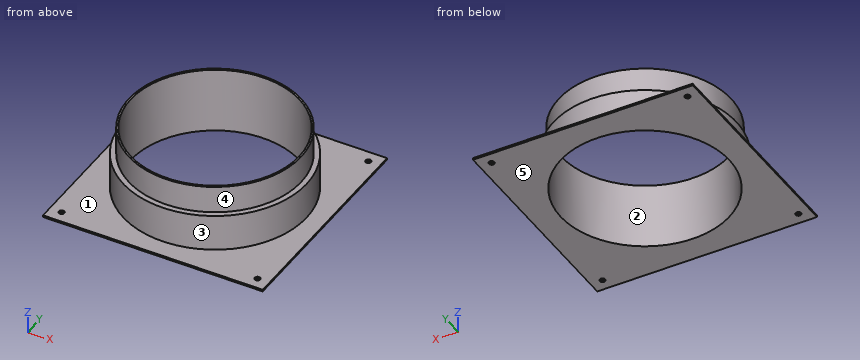
```python
from build123d import *

# Parameters (mm, degrees)
F0_W     = 120
F0_H     = 120
F1_DEPTH = 1
F2_R     = 50
F3_DEPTH = 20
F4_R     = 47
F5_DEPTH = 15
F6_R     = 46
F7_DEPTH = 56.8
F8_R     = 1.5
F9_DEPTH = 25


with BuildPart() as f1:
    # F0 (on Top) → F1 (new body)
    with BuildSketch(Plane.XY):
        Rectangle(F0_W, F0_H)
    extrude(amount=F1_DEPTH)

    # F2 (on face) → F3 (join)
    with BuildSketch(Plane.XY.offset(1)):
        Circle(F2_R)
    extrude(amount=F3_DEPTH)

    # F4 (on face) → F5 (join)
    with BuildSketch(Plane.XY.offset(21)):
        Circle(F4_R)
    extrude(amount=F5_DEPTH)

    # F6 (on face) → F7 (cut)
    with BuildSketch(Plane.XY.offset(36)):
        Circle(F6_R)
    extrude(amount=-F7_DEPTH, mode=Mode.SUBTRACT)

    # F8 (on face) → F9 (cut)
    with BuildSketch(Plane.XY.offset(1)):
        with Locations((-53.5, -53.5)):
            Circle(F8_R)
        with Locations((53.5, -53.5)):
            Circle(F8_R)
        with Locations((-53.5, 53.5)):
            Circle(F8_R)
        with Locations((53.5, 53.5)):
            Circle(F8_R)
    extrude(amount=-F9_DEPTH, mode=Mode.SUBTRACT)


solid = f1.part
```
The listing builds one solid part. Answer for the finished solid, in the listing's coordinates (mm). Face numbers are marked on the shaded views. A direction names the side the tool comes from. Give positions to 0.01 mm unless a question says otherwise; leave off trailing zeros. Order: outer loops, then holes, each group sorted by start corner. A loop starts at its lowest first (then second) coordinate and runs counter-clockwise, first axis right, second up.
1) Find section A-A on y = 53.5. Write down the section's boundary in (x, z), then the cut area to 3 significant figures.
Reported:
outline: (-60, 0) - (-55, 0) - (-55, 1) - (-60, 1) - close; (-52, 0) - (52, 0) - (52, 1) - (-52, 1) - close; (55, 0) - (60, 0) - (60, 1) - (55, 1) - close
area: 114 mm2
2) Find section B-B on x = 0. Write down the section's boundary in (y, z).
Reported:
outline: (-60, 0) - (-46, 0) - (-46, 36) - (-47, 36) - (-47, 21) - (-50, 21) - (-50, 1) - (-60, 1) - close; (46, 0) - (60, 0) - (60, 1) - (50, 1) - (50, 21) - (47, 21) - (47, 36) - (46, 36) - close
3) Find section D-D on y = -23. Write down the section's boundary in (x, z).
Reported:
outline: (-60, 0) - (-39.84, 0) - (-39.84, 36) - (-40.99, 36) - (-40.99, 21) - (-44.4, 21) - (-44.4, 1) - (-60, 1) - close; (39.84, 0) - (60, 0) - (60, 1) - (44.4, 1) - (44.4, 21) - (40.99, 21) - (40.99, 36) - (39.84, 36) - close
4) Determine the mould class of the marked faces 1, 2 and 3 for opening direction X: pulls with the +X half, pulls with the -X half, needs draft (parallel to the pull), parting line crosses it, or undercut.
Reported:
face 1: needs draft
face 2: undercut
face 3: parting line crosses it
5) Consider line 1 along Y through (x, z) = (-53.5, 0.35); line 2 along Z through (x, y) = (49, 26); line 3 along Y through (x, z) = (0, 26). Determine where each line is inside the solid, lowest interval first.
Reported:
line 1: y = -60 to -55, -52 to 52, 55 to 60
line 2: z = 0 to 1
line 3: y = -47 to -46, 46 to 47
6) For the marked faces 4 and 5, determine the directions among +Z, -Z, +X, -X, +Y, -Y from which every point of the face is accessible in a straight line to the end or side of a thin tool.
Reported:
face 4: +Z
face 5: -Z, +X, -X, +Y, -Y
7) Given P1, Ø8, axis at y = -34.5, z = 26.5, coming from the +X side; P2, Ø1.5, axis at y = 29, z = 24, coming from the +X side; P3, Ø1.8, axis at x = -53.5, y = -53.5, coming from the -Z side; P4, Ø3.5, axis at x = 53.5, y = -53.5, coming from the +Z side, each flat-ended and moving along its own axis, determine where each tip first touches the part or whether it passes through.
Reported:
P1: stops at x = 35.76
P2: stops at x = 37.56
P3: passes through
P4: stops at z = 1
